from build123d import *

# Parameters (mm, degrees)
F2_R     = 5.777347
F3_DEPTH = 87.884
F4_R     = 4.634266
F4_R_2   = 4.772292
F4_R_3   = 6.047266
F5_DEPTH = 25.4


with BuildPart() as f1:
    # F0 (on Front) → F1 (revolve)
    with BuildSketch(Plane.XZ):
        with BuildLine():
            Line((0, 61.108096), (0, 0))
            Line((0, 0), (31.088113, 0))
            ThreePointArc((31.088113, 0), (34.053969, 2.04172), (33.205369, 5.540978))
            Line((33.205369, 5.540978), (14.640065, 13.701916))
            ThreePointArc((14.640065, 13.701916), (13.181096, 14.998702), (12.756515, 16.903952))
            Line((12.756515, 16.903952), (8.78591, 67.355268))
            Line((8.78591, 67.355268), (6.247173, 67.355268))
            ThreePointArc((6.247173, 67.355268), (4.417418, 62.93785), (0, 61.108096))
        make_face()
    revolve(axis=Axis((0, 0, 30.554048), (0, 0, 1)))

    # F2 (on face) → F3 (cut)
    with BuildSketch(Plane(origin=(0, 0, 0), x_dir=(1, 0, 0), z_dir=(0, 0, -1))):
        Circle(F2_R)
    extrude(amount=-F3_DEPTH, mode=Mode.SUBTRACT)

    # F4 (on face) → F5 (cut)
    with BuildSketch(Plane(origin=(0, 0, 0), x_dir=(1, 0, 0), z_dir=(0, 0, -1))):
        with Locations((9.536076, 22.793546)):
            Circle(F4_R)
        with Locations((-11.861948, 21.630611)):
            Circle(F4_R_2)
        with Locations((0, -22.560958)):
            Circle(F4_R_3)
    extrude(amount=-F5_DEPTH, mode=Mode.SUBTRACT)


solid = f1.part
Could you check a few things on this model? Use its own coordinates, in mm. Round coordinates to 2 decimals unless told otherwise and drop trailing zeros. Order: outer loops, then holes, each group sorted by start corner. A loop starts at its lowest first (then second) coordinate and runs counter-clockwise, first axis right, second up.
(1) Imagine slicing it at C-C (z = 19). Write out the boundary of the cut face in (x, y), plus the area to 3 significant figures.
Response values:
outline: circle Ø25.18 at (0, 0); hole circle Ø11.55 at (0, 0)
area: 393 mm2
(2) Please list where these lines run through material, in increasing order: line 1 along Y through (x, z) = (0, 6); line 2 along Y through (x, z) = (0, 10); line 3 along Y through (x, z) = (-4.5, 61.5).
Response values:
line 1: y = -32.16 to -5.78, 5.78 to 16.51, 28.61 to 32.16
line 2: y = -23.06 to -5.78, 5.78 to 16.51
line 3: y = -8.08 to -3.62, 3.62 to 8.08
(3) Imagine slicing it at B-B (x = 0). Count the separate pieces of the cut face and the enclosed holes in it, plus the area to 3 significant figures.
Response values:
separate pieces: 3
enclosed holes: 0
area: 1,030 mm2
(4) Imagine slicing it at A-A (z = 44). Write out the boundary of the cut face in (x, y).
Response values:
outline: circle Ø21.25 at (0, 0); hole circle Ø11.55 at (0, 0)
(5) I'm going to push flat-ended pins straight in: pin 1 (7.5 mm diameter, centred on x = 0, y = 22.56, fed in from -Z); pin 2 (12 mm diameter, centred on y = -11, z = 53.5, fed in from -X); pin 3 (3 mm diameter, centred on x = 3.5, z = 15, fed in from -Y); pin 4 (12.5 mm diameter, centred on x = -11.86, y = -21.63, fed in from +Z). Where does each tip first touch, or does it pass through?
Response values:
pin 1: passes through
pin 2: stops at x = -8.56
pin 3: stops at y = -14.71
pin 4: stops at z = 12.04
(6) If we mould it in two halves opening along X, with no side actions, what happens to faces 1 (the cylindrical face through (-0.75, -5.73, 32.03)), 2 (the flat face through (0, -6, 0)), 3 (the conical face through (-10.733, 0.472, 42.483))? For each: released by +X, released by -X, zero draft, split by the parting line, or undercut.
Response values:
face 1: undercut
face 2: zero draft
face 3: split by the parting line
